Can you work these out from the model? Positions are in its coordinate system, mm. Face numbers are marked on the shaded views. A direction names the side the tool comes from. Give positions to 0.01 mm unless a question says otherwise; leave off trailing zeros. Write each loop counter-clockwise with the first axis right and the second up, starting at its lowest first coordinate (ties: lowest second). Pieces come first, ordered by that corner, then holes. Notation, with made-up numbers: (83.5, 67) -> (139.5, 67) arc R13 cw to (139.5, 91) -> close; hole circle Ø8 at (60.25, 2.5). An arc over 180 degrees is marked (long way). Answer as CSV lines item,"result". Start each with the question number.
1. I need wall thicknesses on line 1 (Z direction, x = -10, y = 0); line 2 (Y direction, x = -4.65, z = 10); line 3 (Y direction, x = -2.5, z = 7) (3 decimals). Which ranges of each line are inside material? Lowest first, please. Write a range as [from, to].
2. I'm going to push flat-ended pins straight in: P1, Ø0.9, axis at x = 2, y = 3.5, coming from the +Z side; P2, Ø4, axis at y = -2.5, z = -3, coming from the +X side; P3, Ø0.8, axis at x = -7.5, y = -0.5, coming from the -Z side (3 decimals). Where does each tip first touch, or does it pass through?
3. If we section it at B-B on z = -0.5: Write out the boundary of the cut face in (x, y), plus the area to 3 significant figures.
4. If we section it at D-D on y = -4.5: Write out the boundary of the cut face in (x, z).
5. If we mould it in two halves opening along Y, with no side actions, what happens to the marked faces 1, 2 and 3? For each: pulls with the +Y half, pulls with the -Y half, needs draft (parallel to the pull), parting line crosses it, or undercut.
6. If we section it at C-C on x = -4: Write out the boundary of the cut face in (y, z).
7. On a 3-axis mill with a long thin cutter (end or side, diameter ignored), from which of +Z, -Z, +X, -X, +Y, -Y can I reach the whole of each face in a straight line? I mean the marked faces 4, 5 and 6. Say none if no direction works.
8. If we section it at A-A on y = 0: Count the separate pieces of the cut face and the enclosed holes in it, plus the area to 3 significant figures.
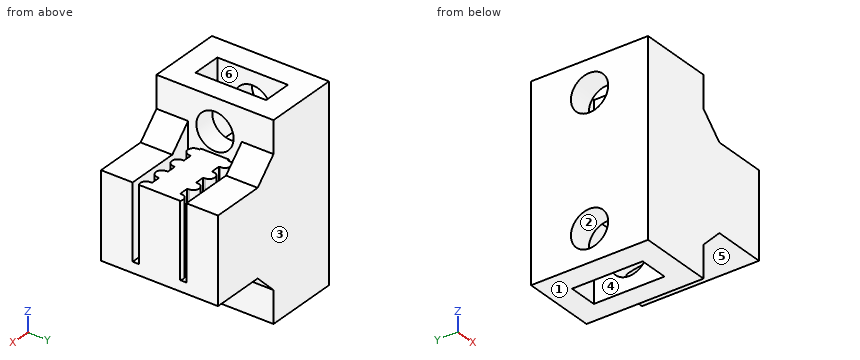
```python
from build123d import *

# Parameters (mm, degrees)
SKETCH_1_W          = 7
SKETCH_1_H          = 11
EXTRUDE_1_DEPTH     = 8
CUT_EXTRUDE_1_DEPTH = 7
SKETCH_3_W          = 18
SKETCH_3_H          = 11
SKETCH_3_R          = 1.75
EXTRUDE_2_DEPTH     = 7
CUT_EXTRUDE_START   = -2
SKETCH_5_W          = 0.875
SKETCH_5_H          = 2.65
SKETCH_5_R          = 1.75
CUT_EXTRUDE_3_DEPTH = 2.75
CHAMFER_1_SIZE      = 2


with BuildPart() as part:
    # Эскиз1 → Бобышка-Вытянуть1 (new body)
    with BuildSketch(Plane.XY):
        Rectangle(SKETCH_1_W, SKETCH_1_H)
    extrude(amount=EXTRUDE_1_DEPTH)

    # Эскиз2 → Вырез-Вытянуть1 (cut)
    with BuildSketch(Plane.XY.offset(8)):
        with BuildLine():
            Line((-3.5, 2.525), (-3.5, 1.325))
            Line((-3.5, 1.325), (-3.35, 1.325))
            Line((-3.35, 1.325), (-3.331582316, 1.475))
            ThreePointArc((-3.331582316, 1.475), (-2.781582316, 2.025), (-2.231582316, 1.475))
            Line((-2.231582316, 1.475), (-2.213164632, 1.325))
            Line((-2.213164632, 1.325), (-1.35, 1.325))
            Line((-1.35, 1.325), (-1.331582316, 1.475))
            ThreePointArc((-1.331582316, 1.475), (-0.781582316, 2.025), (-0.231582316, 1.475))
            Line((-0.231582316, 1.475), (-0.213164632, 1.325))
            Line((-0.213164632, 1.325), (0.65, 1.325))
            Line((0.65, 1.325), (0.668417684, 1.475))
            ThreePointArc((0.668417684, 1.475), (1.218417684, 2.025), (1.768417684, 1.475))
            Line((1.768417684, 1.475), (1.786835368, 1.325))
            Line((1.786835368, 1.325), (2.65, 1.325))
            Line((2.65, 1.325), (2.668417684, 1.475))
            ThreePointArc((2.668417684, 1.475), (2.946728775, 1.953210348), (3.5, 1.947452537))
            Line((3.5, 1.947452537), (3.5, 2.525))
            Line((3.5, 2.525), (-3.5, 2.525))
        make_face()
        with BuildLine():
            Line((-3.35, -1.325), (-3.5, -1.325))
            Line((-3.5, -1.325), (-3.5, -2.525))
            Line((-3.5, -2.525), (3.5, -2.525))
            Line((3.5, -2.525), (3.5, -1.947452537))
            ThreePointArc((3.5, -1.947452537), (2.946728775, -1.953210348), (2.668417684, -1.475))
            Line((2.668417684, -1.475), (2.65, -1.325))
            Line((2.65, -1.325), (1.786835368, -1.325))
            Line((1.786835368, -1.325), (1.768417684, -1.475))
            ThreePointArc((1.768417684, -1.475), (1.218417684, -2.025), (0.668417684, -1.475))
            Line((0.668417684, -1.475), (0.65, -1.325))
            Line((0.65, -1.325), (-0.213164632, -1.325))
            Line((-0.213164632, -1.325), (-0.231582316, -1.475))
            ThreePointArc((-0.231582316, -1.475), (-0.781582316, -2.025), (-1.331582316, -1.475))
            Line((-1.331582316, -1.475), (-1.35, -1.325))
            Line((-1.35, -1.325), (-2.213164632, -1.325))
            Line((-2.213164632, -1.325), (-2.231582316, -1.475))
            ThreePointArc((-2.231582316, -1.475), (-2.781582316, -2.025), (-3.331582316, -1.475))
            Line((-3.331582316, -1.475), (-3.35, -1.325))
        make_face()
    extrude(amount=-CUT_EXTRUDE_1_DEPTH, mode=Mode.SUBTRACT)

    # Эскиз3 → Бобышка-Вытянуть2 (add)
    with BuildSketch(Plane.ZY.offset(3.5)):
        with Locations((4, 0)):
            Rectangle(SKETCH_3_W, SKETCH_3_H)
        with Locations((10, 0)):
            Circle(SKETCH_3_R, mode=Mode.SUBTRACT)
        with Locations((-2, 0)):
            Circle(SKETCH_3_R, mode=Mode.SUBTRACT)
    extrude(amount=EXTRUDE_2_DEPTH)

    # Эскиз5 → Вырез-Вытянуть3 (cut)
    # profile 1 of 5: a face of its own
    with BuildSketch(Plane(origin=(-3.5, 0, 0), x_dir=(0, 0, -1), z_dir=(1, 0, 0)).offset(CUT_EXTRUDE_START)):
        Polygon((2, 3.319764048), (4.875, 1.659882024), (4.875, -1.659882024), (2, -3.319764048), (-0.875, -1.659882024), (-0.875, 1.659882024), align=None)
    # profile 2 of 5: a face of its own
    with BuildSketch(Plane(origin=(-3.5, 0, 0), x_dir=(0, 0, -1), z_dir=(1, 0, 0)).offset(CUT_EXTRUDE_START)):
        Polygon((5, 3.319764048), (5, -3.319764048), (2, -3.319764048), (4.875, -1.659882024), (4.875, 1.659882024), (2, 3.319764048), align=None)
    # profile 3 of 5: a face of its own
    with BuildSketch(Plane(origin=(-3.5, 0, 0), x_dir=(0, 0, -1), z_dir=(1, 0, 0)).offset(CUT_EXTRUDE_START)):
        with Locations((-7.5625, 0)):
            Rectangle(SKETCH_5_W, SKETCH_5_H)
    # profile 4 of 5: a face of its own
    with BuildSketch(Plane(origin=(-3.5, 0, 0), x_dir=(0, 0, -1), z_dir=(1, 0, 0)).offset(CUT_EXTRUDE_START)):
        Polygon((-7.125, 1.659882024), (-10, 3.319764048), (-12.875, 1.659882024), (-12.875, -1.659882024), (-10, -3.319764048), (-7.125, -1.659882024), (-7.125, -1.325), (-8, -1.325), (-8, 1.325), (-7.125, 1.325), align=None)
        with Locations((-10, 0)):
            Circle(SKETCH_5_R, mode=Mode.SUBTRACT)
    # profile 5 of 5: a face of its own
    with BuildSketch(Plane(origin=(-3.5, 0, 0), x_dir=(0, 0, -1), z_dir=(1, 0, 0)).offset(CUT_EXTRUDE_START)):
        Polygon((-12.875, 1.659882024), (-10, 3.319764048), (-13, 3.319764048), (-13, -3.319764048), (-10, -3.319764048), (-12.875, -1.659882024), align=None)
    extrude(amount=-CUT_EXTRUDE_3_DEPTH, mode=Mode.SUBTRACT)

    # Фаска1
    # the kernel refuses this chamfer: 2 mm, written as the material it adds along each edge
    with BuildSketch(Plane(origin=(-3.5, 5.5, 8), x_dir=(1, 0, 0), z_dir=(0, -1, 0)), Plane(origin=(-3.5, -2.525, 8), x_dir=(1, 0, 0), z_dir=(0, -1, 0))) as chamfer_1_piece_1:
        Polygon((CHAMFER_1_SIZE, 0), (0, CHAMFER_1_SIZE), (0, 0), align=None)
    extrude(amount=2.975)
    with BuildSketch(Plane(origin=(-3.5, 10.643365976, 8), x_dir=(1, 0, 0), z_dir=(0, -1, 0))) as chamfer_1_piece_2_section:
        Polygon((CHAMFER_1_SIZE, 0), (0, CHAMFER_1_SIZE), (0, 0), align=None)
    chamfer_1_piece_2 = extrude(amount=13.261731952, mode=Mode.PRIVATE)
    chamfer_1_piece_2 = split(chamfer_1_piece_2, bisect_by=Plane(origin=(-3.5, -2.525, 8), z_dir=(0, -1, 0)), keep=Keep.TOP, mode=Mode.PRIVATE)
    add(chamfer_1_piece_2)
    with BuildSketch(Plane(origin=(-3.5, 2.618365976, 8), x_dir=(1, 0, 0), z_dir=(0, -1, 0))) as chamfer_1_piece_3_section:
        Polygon((CHAMFER_1_SIZE, 0), (0, CHAMFER_1_SIZE), (0, 0), align=None)
    chamfer_1_piece_3 = extrude(amount=13.261731952, mode=Mode.PRIVATE)
    chamfer_1_piece_3 = split(chamfer_1_piece_3, bisect_by=Plane(origin=(-3.5, 2.525, 8), z_dir=(0, 1, 0)), keep=Keep.TOP, mode=Mode.PRIVATE)
    add(chamfer_1_piece_3)
    with BuildSketch(Plane(origin=(-3.5, 5.5, 0), x_dir=(0, 0, -1), z_dir=(0, -1, 0))) as chamfer_1_piece_4_section:
        Polygon((CHAMFER_1_SIZE, 0), (0, CHAMFER_1_SIZE), (0, 0), align=None)
    chamfer_1_piece_4 = extrude(amount=11, mode=Mode.PRIVATE)
    chamfer_1_piece_4 = chamfer_1_piece_4 - Plane(origin=(-3.5, 0, -2), x_dir=(0, 0, 1), z_dir=(1, 0, 0)) * Cylinder(1.75, 30, mode=Mode.PRIVATE)
    add(chamfer_1_piece_4)


solid = part.part
```
Computed values:
1,line 1,"z = [-5, -3.75], [-0.25, 8.25], [11.75, 13]"
1,line 2,"y = [-5.5, -1.75], [1.75, 5.5]"
1,line 3,"y = [-5.5, -2.525], [-1.947, 1.947], [2.525, 5.5]"
2,P1,"stops at z = 8"
2,P2,"stops at x = -2.5"
2,P3,"stops at z = 0.875"
3,outline,"(-10.5, -5.5) -> (-2, -5.5) -> (-2, -0.9) -> (-5.5, -0.9) -> (-5.5, -2.45) -> (-8.25, -2.45) -> (-8.25, -0.9) -> (-10.5, -0.9) -> close; (-10.5, 0.9) -> (-8.25, 0.9) -> (-8.25, 2.45) -> (-5.5, 2.45) -> (-5.5, 0.9) -> (-2, 0.9) -> (-2, 5.5) -> (-10.5, 5.5) -> close"
3,area,"69.6 mm2"
4,outline,"(-10.5, -5) -> (-3.5, -5) -> (-3.5, -2) -> (-1.5, 0) -> (3.5, 0) -> (3.5, 8) -> (-1.5, 8) -> (-3.5, 10) -> (-3.5, 13) -> (-10.5, 13) -> close"
5,face 1,"needs draft"
5,face 2,"undercut"
5,face 3,"pulls with the +Y half"
6,outline,"(-5.5, -5) -> (5.5, -5) -> (5.5, 13) -> (-5.5, 13) -> close; hole circle Ø3.5 at (0, -2); hole circle Ø3.5 at (0, 10)"
7,face 4,"-Z"
7,face 5,"-Z, +X, +Y, -Y"
7,face 6,"+Z"
8,separate pieces,"5"
8,enclosed holes,"0"
8,area,"120 mm2"
